Source: CAD feature listing. Evaluate the final solid. Frame: model axes, mm. Face numbers are marked on the shaded views. A direction names the side the tool comes from. Give positions to 0.01 mm unless a question says otherwise; leave off trailing zeros. Order: outer loops, then holes, each group sorted by start corner. A loop starts at its lowest first (then second) coordinate and runs counter-clockwise, first axis right, second up. Notation, with made-up numbers: (0.5, 71.5) - (23.5, 71.5) arc R14 cw to (23.5, 94.5) - close; hole circle Ø8 at (-31, 84). An arc over 180 degrees is marked (long way). Answer as CSV lines item,"result".
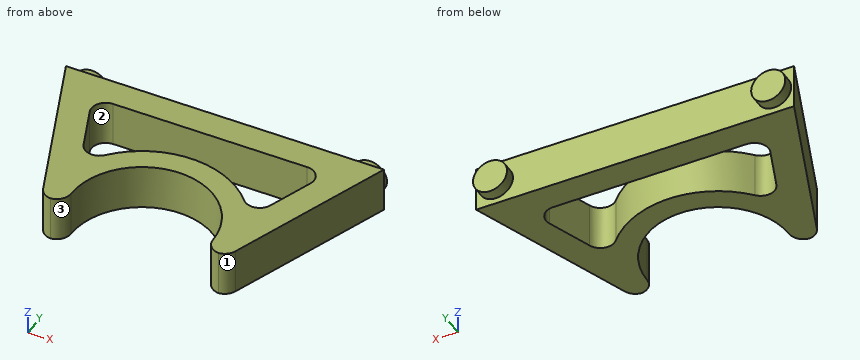
```python
from build123d import *

# Parameters (mm, degrees)
BOSS_EXTRUDE1_DEPTH = 8
CUT_EXTRUDE1_DEPTH  = 43.16930163
FILLET1_R           = 2.5
SKETCH3_R           = 3
BOSS_EXTRUDE2_DEPTH = 2


with BuildPart() as part:
    # Sketch1 → Boss-Extrude1 (new body)
    with BuildSketch(Plane.XY):
        with BuildLine():
            Line((-28, 0), (28, 0))
            Line((28, 0), (16.30950643, -30.5))
            Line((16.30950643, -30.5), (12.247448714, -30.5))
            ThreePointArc((12.247448714, -30.5), (0, -15.5), (-12.247448714, -30.5))
            Line((-12.247448714, -30.5), (-16.30950643, -30.5))
            Line((-16.30950643, -30.5), (-28, 0))
        make_face()
    extrude(amount=BOSS_EXTRUDE1_DEPTH)

    # Sketch2 → Cut-Extrude1 (cut, through all)
    with BuildSketch(Plane.XY.offset(8)):
        with BuildLine():
            Line((-20.728819868, -5), (-14.748606624, -20.602121746))
            ThreePointArc((-14.748606624, -20.602121746), (0, -11.5), (14.748606624, -20.602121746))
            Line((14.748606624, -20.602121746), (20.728819868, -5))
            Line((20.728819868, -5), (-20.728819868, -5))
        make_face()
    extrude(amount=-CUT_EXTRUDE1_DEPTH, mode=Mode.SUBTRACT)

    # Fillet1
    # the kernel refuses this fillet: 2.5 mm, written as the material it adds along each edge
    with BuildSketch(Plane(origin=(14.748606624, -20.602121746, 8), x_dir=(0.35790469832996064, 0.9337581201324783, 0), z_dir=(0, 0, -1))) as fillet1_piece_1:
        with BuildLine():
            CenterArc((4.743679492, -2.5), FILLET1_R, 90, 116.993489573)
            ThreePointArc((2.516034231, -3.634723133), (1.38029262, -1.732719809), (0, 0))
            Line((0, 0), (4.743679492, 0))
        make_face()
    extrude(amount=8)
    with BuildSketch(Plane(origin=(20.728819868, -5, 8), x_dir=(-0.35790469832996097, -0.9337581201324782, 0), z_dir=(0, 0, -1))) as fillet1_piece_2:
        with BuildLine():
            CenterArc((FILLET1_R * 1.4542360265, FILLET1_R), FILLET1_R, 159.028427988, 110.971572012)
            Line((FILLET1_R * 0.520477906364, FILLET1_R * 1.35790469833), (0, 0))
            Line((0, 0), (FILLET1_R * 1.4542360265, 0))
        make_face()
    extrude(amount=8)
    with BuildSketch(Plane(origin=(-20.728819868, -5, 8), x_dir=(0.35790469832996097, -0.9337581201324782, 0), z_dir=(0, 0, -1))) as fillet1_piece_3:
        with BuildLine():
            CenterArc((FILLET1_R * 1.4542360265, -FILLET1_R), FILLET1_R, 90, 110.971572012)
            Line((FILLET1_R * 0.520477906364, -FILLET1_R * 1.35790469833), (0, 0))
            Line((0, 0), (FILLET1_R * 1.4542360265, 0))
        make_face()
    extrude(amount=8)
    with BuildSketch(Plane(origin=(-14.748606624, -20.602121746, 8), x_dir=(0.5640537125230959, 0.8257380997561593, 0), z_dir=(0, 0, -1))) as fillet1_piece_4:
        with BuildLine():
            CenterArc((4.755486169, -2.477467743), FILLET1_R, 97.698333221, 116.993489574)
            Line((2.69992297, -3.900373197), (0, 0))
            ThreePointArc((0, 0), (2.210296389, -0.148712899), (4.420592777, 0))
        make_face()
    extrude(amount=8)
    # the kernel refuses this fillet: 2.5 mm, written as the material it takes off along each edge
    with BuildSketch(Plane(origin=(12.247448714, -30.5, -6.881378215), x_dir=(1, 0, 0), z_dir=(0, 0, 1))) as fillet1_2_piece_1:
        with BuildLine():
            CenterArc((2.752551286, 2.5), FILLET1_R, 180, 90)
            ThreePointArc((0.252551286, 2.5), (0.189253199, 1.243637975), (0, 0))
            Line((0, 0), (2.752551286, 0))
        make_face()
    extrude(amount=21.76275643, mode=Mode.SUBTRACT)
    with BuildSketch(Plane(origin=(16.30950643, -30.5, -4.297789276), x_dir=(0.3579046983299623, 0.9337581201324777, 0), z_dir=(0, 0, 1))) as fillet1_2_piece_2:
        with BuildLine():
            CenterArc((FILLET1_R * 0.687646284221, FILLET1_R), FILLET1_R, 200.971572012, 69.028427988)
            Line((-FILLET1_R * 0.246111835912, FILLET1_R * 0.64209530167), (0, 0))
            Line((0, 0), (FILLET1_R * 0.687646284221, 0))
        make_face()
    extrude(amount=16.595578553, mode=Mode.SUBTRACT)
    with BuildSketch(Plane(origin=(-12.247448714, -30.5, -6.881378215), x_dir=(-1, 0, 0), z_dir=(0, 0, 1))) as fillet1_2_piece_3:
        with BuildLine():
            CenterArc((2.752551286, -2.5), FILLET1_R, 90, 90)
            ThreePointArc((0.252551286, -2.5), (0.189253199, -1.243637975), (0, 0))
            Line((0, 0), (2.752551286, 0))
        make_face()
    extrude(amount=21.76275643, mode=Mode.SUBTRACT)
    with BuildSketch(Plane(origin=(-16.30950643, -30.5, -4.297789276), x_dir=(-0.3579046983299605, 0.9337581201324784, 0), z_dir=(0, 0, 1))) as fillet1_2_piece_4:
        with BuildLine():
            CenterArc((FILLET1_R * 0.687646284221, -FILLET1_R), FILLET1_R, 90, 69.028427988)
            Line((-FILLET1_R * 0.246111835912, -FILLET1_R * 0.64209530167), (0, 0))
            Line((0, 0), (FILLET1_R * 0.687646284221, 0))
        make_face()
    extrude(amount=16.595578553, mode=Mode.SUBTRACT)

    # Sketch3 → Boss-Extrude2 (add)
    with BuildSketch(Plane(origin=(0, 0, 0), x_dir=(1, 0, 0), z_dir=(0, 1, 0))):
        with Locations(Location((-24.5, -4, 0), (0, 0, 180))):
            Circle(SKETCH3_R)
        with Locations(Location((24.5, -4, 0), (0, 0, 180))):
            Circle(SKETCH3_R)
    extrude(amount=BOSS_EXTRUDE2_DEPTH)


solid = part.part
```
(1) Cut plane D-D (x = 24.5). Return loops of the section in (y, z).
Completed:
outline,"(-9.13, 0) - (0, 0) - (0, 1) - (2, 1) - (2, 7) - (0, 7) - (0, 8) - (-9.13, 8) - close"
(2) Access query for the marked faces 1, 2 and 3. Directions: +Z, -Z, +X, -X, +Y, -Y. A direction counts if a zero-diameter tool reaches every point of the face in a straight line with its end or side. Return the directions, or none.
Completed:
face 1,"+Z, -Z, +X, -Y"
face 2,"+Z, -Z"
face 3,"+Z, -Z, -Y"
(3) Contact query for flat-ended pins moving along their axis: pin 1 (4 mm diameter, centred on x = 11, z = 7, fed in from +Y); pin 2 (1.5 mm diameter, centred on x = -8, z = 4, fed in from -Y); pin 3 (1 mm diameter, centred on x = 4.5, z = 1.5, fed in from -Y). Output: stop coordinate, or through.
Completed:
pin 1,"y = 0"
pin 2,"y = -19.07"
pin 3,"y = -16.54"
(4) Cut plane B-B (y = -19). Return loops of the section in (x, z), then the cut area to 3 significant figures.
Completed:
outline,"(-20.72, 0) - (-8.67, 0) - (-8.67, 8) - (-20.72, 8) - close; (8.67, 0) - (20.72, 0) - (20.72, 8) - (8.67, 8) - close"
area,"193 mm²"
(5) Ray query, line 1 (Y direction, x = 0.5, z = 5.75); line 2 (X direction, y = -15, z = 3.25); line 3 (Y direction, x = 5.5, z = 7). Return the intervals inside material, ascending. Write a range as from..to.
Completed:
line 1,"-15.51..-11.51, -5..0"
line 2,"-22.25..-16.9, -10.16..10.16, 16.9..22.25"
line 3,"-16.78..-12.44, -5..0"
(6) Cut plane A-A (x = 0). Return loops of the section in (y, z).
Completed:
outline,"(-15.5, 0) - (-11.5, 0) - (-11.5, 8) - (-15.5, 8) - close; (-5, 0) - (0, 0) - (0, 8) - (-5, 8) - close"
(7) Cut plane C-C (z = 4). Return loops of the section in (x, y).
Completed:
outline,"(-28, 0) - (-16.92, -28.89) arc R2.5 ccw to (-14.8, -30.49) arc R2.5 ccw to (-12.5, -28) arc R12.5 cw to (12.5, -28) arc R2.5 ccw to (14.8, -30.49) arc R2.5 ccw to (16.92, -28.89) - (28, 0) - (27.5, 0) - (27.5, 2) - (21.5, 2) - (21.5, 0) - (-21.5, 0) - (-21.5, 2) - (-27.5, 2) - (-27.5, 0) - close; hole (-19.43, -8.39) - (-16.45, -16.17) arc R2.5 ccw to (-12.26, -16.95) arc R16.5 cw to (12.26, -16.95) arc R2.5 ccw to (16.45, -16.17) - (19.43, -8.39) arc R2.5 ccw to (17.09, -5) - (-17.09, -5) arc R2.5 ccw to start"
